```python
from build123d import *

# Parameters (mm, degrees)
BOSS_EXTRU_1_DEPTH = 2
ESQUISSE3_W        = 14.4
ESQUISSE3_H        = 8.4
ESQUISSE3_W_2      = 10.4
ESQUISSE3_H_2      = 4.4
BOSS_EXTRU_3_DEPTH = 15
D_POUILLE3_ANGLE   = 2


with BuildPart() as part:
    # Esquisse1 → Boss.-Extru.1 (new body)
    with BuildSketch(Plane.XY):
        Polygon((16.568542495, -40), (40, -16.568542495), (40, 16.568542495), (16.568542495, 40), (-16.568542495, 40), (-40, 16.568542495), (-40, -16.568542495), (-16.568542495, -40), align=None)
    extrude(amount=BOSS_EXTRU_1_DEPTH)

    # Esquisse3 → Boss.-Extru.3 (add)
    with BuildSketch(Plane.XZ.offset(40)):
        with Locations((0, -2.3)):
            Rectangle(ESQUISSE3_W, ESQUISSE3_H)
        with Locations((0, -2.3)):
            Rectangle(ESQUISSE3_W_2, ESQUISSE3_H_2, mode=Mode.SUBTRACT)
    extrude(amount=-BOSS_EXTRU_3_DEPTH)

    # Dépouille3
    d_pouille3_faces = [part.faces().sort_by_distance(p)[0] for p in [
        (0, -32.5, -0.1),
        (-5.2, -32.5, -2.3),
        (0, -32.5, -4.5),
        (5.2, -32.5, -2.3),
    ]]
    draft(d_pouille3_faces, Plane(origin=(-16.568542495, -40, 2), x_dir=(-1, 0, 0), z_dir=(0, -1, 0)), D_POUILLE3_ANGLE)


solid = part.part
```
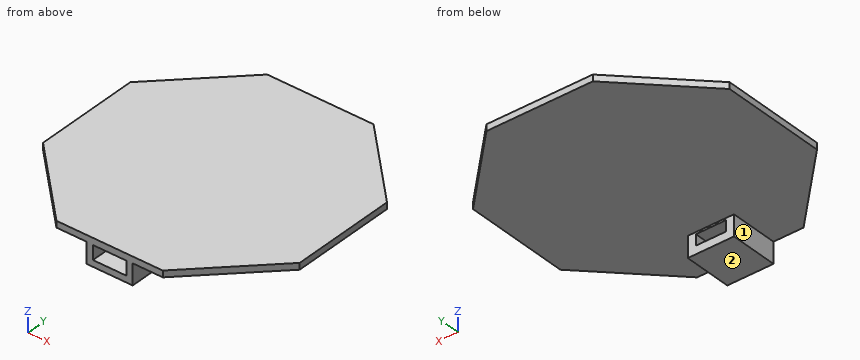
The listing builds one solid part. Answer for the finished solid, in the listing's coordinates (mm). Face numbers are marked on the shaded views. A direction names the side the tool comes from. Give positions to 0.01 mm unless a question says otherwise; leave off trailing zeros. Order: outer loops, then holes, each group sorted by start corner. A loop starts at its lowest first (then second) coordinate and runs counter-clockwise, first axis right, second up. Notation, with made-up numbers: (55.5, 27) -> (92.5, 27) arc R27 cw to (92.5, 46) -> close; hole circle Ø4 at (-38, 48). An arc over 180 degrees is marked (long way). Answer as a JSON object with one key per item and string values. Group by question number.
Item 1: The part is cut by section C-C on z = 1. Write down the section's boundary in (x, y), and give its area (3 significant figures).
Item 2: The part is cut by section B-B on z = -3. Write down the section's boundary in (x, y), and give its area (3 significant figures).
Item 3: The part is cut by section D-D on y = -29.5. Write down the section's boundary in (x, z).
Item 4: Consider L1, parallel to Z at x = 9, y = -32; L2, parallel to X at y = -29, z = -1.5; L3, parallel to Y at x = -36, z = 1.5. Determine where each line is inside the solid, lowest interval first. Write a range as from..to.
Item 5: A tool of negligible diameter and unlimited length cuts with its end or side. For the marked faces 1 and 2, from which of +Z, -Z, +X, -X, +Y, -Y can it reach the whole face along a straight path? Write none if from no direction.
Item 6: Flat-ended cylindrical pins translate along their axes: pin 1 (1 mm diameter, centred on x = 31.5, y = -14, fed in from -Z); pin 2 (3 mm diameter, centred on x = -3.5, z = -2, fed in from +Y); pin 3 (2 mm diameter, centred on y = -29.5, z = -2.5, fed in from -X). Find the tip coordinate at first contact, or state that the pin passes through.
Item 7: The part is cut by section A-A on x = -0.5. Write down the section's boundary in (y, z), and give its area (3 significant figures).
Result set:
{
 "1": {"outline": "(-40, -16.57) -> (-16.57, -40) -> (16.57, -40) -> (40, -16.57) -> (40, 16.57) -> (16.57, 40) -> (-16.57, 40) -> (-40, 16.57) -> close", "area": "5,300 mm²"},
 "2": {"outline": "(-7.2, -40) -> (-5.2, -40) -> (-4.68, -25) -> (-7.2, -25) -> close; (4.68, -25) -> (5.2, -40) -> (7.2, -40) -> (7.2, -25) -> close", "area": "67.9 mm²"},
 "3": {"outline": "(-27.07, 0) -> (-7.2, 0) -> (-7.2, -6.5) -> (7.2, -6.5) -> (7.2, 0) -> (27.07, 0) -> (27.07, 2) -> (-27.07, 2) -> close; hole (-4.83, -4.13) -> (4.83, -4.13) -> (4.83, -0.47) -> (-4.83, -0.47) -> close"},
 "4": {"L1": "0..2", "L2": "-7.2..-4.82, 4.82..7.2", "L3": "-20.57..20.57"},
 "5": {"face 1": "-Z, -X, +Y, -Y", "face 2": "-Z, +X, -X, +Y, -Y"},
 "6": {"pin 1": "z = 0", "pin 2": "y = -25", "pin 3": "x = -7.2"},
 "7": {"outline": "(-40, -6.5) -> (-25, -6.5) -> (-25, -3.98) -> (-40, -4.5) -> close; (-40, -0.1) -> (-25, -0.62) -> (-25, 0) -> (40, 0) -> (40, 2) -> (-40, 2) -> close", "area": "199 mm²"}
}
